```python
from build123d import *

# Parameters (mm, degrees)
SKETCH1_W           = 19.05
SKETCH1_H           = 19.05
BOSS_EXTRUDE1_DEPTH = 5.08
SKETCH2_R           = 8.255
BOSS_EXTRUDE2_DEPTH = 15.24
CUT_EXTRUDE1_DEPTH  = 25.379369352
FILLET1_R           = 2.54
CHAMFER1_SIZE       = 0.508


with BuildPart() as part:
    # Sketch1 → Boss-Extrude1 (new body)
    with BuildSketch(Plane.XY):
        Rectangle(SKETCH1_W, SKETCH1_H)
    extrude(amount=-BOSS_EXTRUDE1_DEPTH)

    # Sketch2 → Boss-Extrude2 (add)
    with BuildSketch(Plane(origin=(0, 0, -5.08), x_dir=(-1, 0, 0), z_dir=(0, 0, -1))):
        with Locations(Location((0, 0, 0), (0, 0, 180))):
            Circle(SKETCH2_R)
    extrude(amount=BOSS_EXTRUDE2_DEPTH)

    # Sketch3 → Cut-Extrude1 (cut, through all)
    with BuildSketch(Plane.XY):
        Polygon((3.666174209, 6.35), (-3.666174209, 6.35), (-7.332348419, 0), (-3.666174209, -6.35), (3.666174209, -6.35), (7.332348419, 0), align=None)
    extrude(amount=-CUT_EXTRUDE1_DEPTH, mode=Mode.SUBTRACT)

    # Fillet1
    fillet1_edges = [part.edges().sort_by_distance(p)[0] for p in [
        (9.525, -9.525, -2.54),
        (-9.525, -9.525, -2.54),
        (-9.525, 9.525, -2.54),
        (9.525, 9.525, -2.54),
    ]]
    fillet(fillet1_edges, radius=FILLET1_R)

    # Chamfer1
    chamfer1_edges = [part.edges().sort_by_distance(p)[0] for p in [
        (5.499261314, 3.175, 0),
        (0, 6.35, 0),
        (-5.499261314, 3.175, 0),
        (-5.499261314, -3.175, 0),
        (0, -6.35, 0),
        (5.499261314, -3.175, 0),
    ]]
    chamfer(chamfer1_edges, length=CHAMFER1_SIZE)


solid = part.part
```
Check sheet for the modelled part. Datum: model origin and axes. Units: mm. A direction names the side the tool comes from. Coordinates: 2 decimals unless noted, no trailing zeros. Order: outer loops, then holes, each group sorted by start corner. A loop starts at its lowest first (then second) coordinate and runs counter-clockwise, first axis right, second up. Notation, with made-up numbers: M 79,24 L 136,24 A13 cw 136,40 Z; hole C -35.75,32 d3. An arc over 180 degrees is marked long. One line per question, with ' | ' between items. Start each with the question number.
Item 1: Sectioned sample at C-C on y = -2.5. Record the cut outline in (x, z) (3 decimals), and give its area (3 significant figures).
Item 2: Material ranges on line 1 (Y direction, x = -0.5, z = -1.25) (3 decimals); line 2 (X direction, y = -2.5, z = -14.5); line 3 (Y direction, x = 6, z = -7.5), recorded low to high.
Item 3: Sectioned sample at A-A on x = 0. Record the cut outline in (y, z) (3 decimals), and give its area (3 significant figures).
Item 4: Access from +Z, -Z, +X, -X, +Y, -Y to the whole of each face (thin tool, end or side, straight path). Record for faces 1 (the flat face through (-9, 0, -5.08)), 2 (the flat face through (-5.688, 3.348, -0.258)), 3 (the flat face through (5.474, -3.219, -10.275)).
Item 5: Mould release check, pull along Y, two halves, no side actions. Record for faces 4 (the cylindrical face through (-8.8, -8.76, -2.58)), 5 (the flat face through (5.688, -3.348, -0.258)), 6 (the flat face through (9.525, 0, -3)): pulls with the +Y half, pulls with the -Y half, needs draft (parallel to the pull), parting line crosses it, or undercut.
Item 6: Sectioned sample at D-D on z = -8.25. Record the cut outline in (x, y) (3 decimals), and give its area (3 significant figures).
Item 7: Gauge pin test, flat ends, axial feed: P1, Ø6, axis at x = 7, z = -16, coming from the +Y side; P2, Ø3.5, axis at x = -1, z = -15, coming from the +Y side (3 decimals); P3, Ø3, axis at x = 4.5, z = -13.5, coming from the +Y side. Record the tip position at first contact, or that the pin passes through.
Item 8: Sectioned sample at B-B on z = -1.5. Record the cut outline in (x, y) (3 decimals), and give its area (3 significant figures).
Answer below:
1) outline: M -9.525,-5.08 L -7.867,-5.08 L -7.867,-20.32 L -5.889,-20.32 L -5.889,-0.508 L -6.476,0 L -9.525,0 Z; M 5.889,-20.32 L 7.867,-20.32 L 7.867,-5.08 L 9.525,-5.08 L 9.525,0 L 6.476,0 L 5.889,-0.508 Z | area: 96.9 mm^2
2) line 1: y = -9.525 to -6.35, 6.35 to 9.525 | line 2: x = -7.87 to -5.89, 5.89 to 7.87 | line 3: y = -5.67 to -2.31, 2.31 to 5.67
3) outline: M -9.525,-5.08 L -8.255,-5.08 L -8.255,-20.32 L -6.35,-20.32 L -6.35,-0.508 L -6.858,0 L -9.525,0 Z; M 6.35,-20.32 L 8.255,-20.32 L 8.255,-5.08 L 9.525,-5.08 L 9.525,0 L 6.858,0 L 6.35,-0.508 Z | area: 90.1 mm^2
4) face 1: -Z | face 2: +Z | face 3: +Z, -Z
5) face 4: pulls with the -Y half | face 5: undercut | face 6: needs draft
6) outline: C 0,0 d16.51; hole M -7.332,0 L -3.666,-6.35 L 3.666,-6.35 L 7.332,0 L 3.666,6.35 L -3.666,6.35 Z | area: 74.4 mm^2
7) P1: stops at y = 7.22 | P2: stops at y = 8.255 | P3: stops at y = 7.69
8) outline: M -9.525,-6.985 A2.54 ccw -6.985,-9.525 L 6.985,-9.525 A2.54 ccw 9.525,-6.985 L 9.525,6.985 A2.54 ccw 6.985,9.525 L -6.985,9.525 A2.54 ccw -9.525,6.985 Z; hole M -7.332,0 L -3.666,-6.35 L 3.666,-6.35 L 7.332,0 L 3.666,6.35 L -3.666,6.35 Z | area: 218 mm^2
